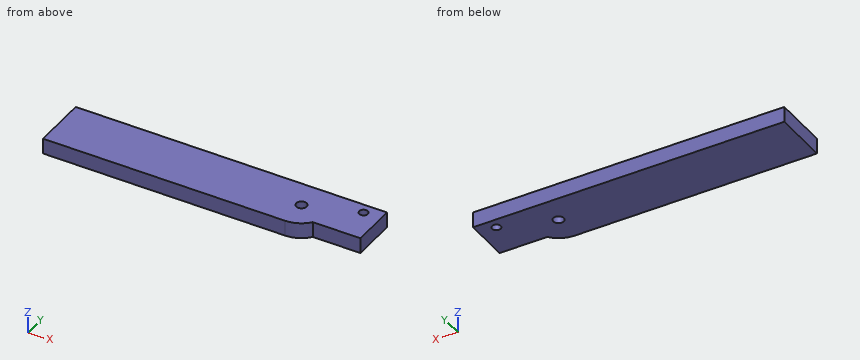
```python
from build123d import *

# Parameters (mm, degrees)
F1_DEPTH = 4.5
F2_D     = 3
F2_DEPTH = 10
F2_TIP   = 0.9012909285
F3_D     = 2.5
F3_DEPTH = 10
F3_TIP   = 0.7510757738


with BuildPart() as f1:
    # F0 (on Top) → F1 (new body)
    with BuildSketch(Plane.XY):
        Polygon((35, -5), (35, 8), (-35, 8), (-35, -8), (35, -8), align=None)
        with BuildLine():
            Line((41.2449979984, -5), (35, -5))
            Line((35, -5), (35, -8))
            ThreePointArc((35, -8), (38.4641016151, -7.2111025509), (41.2449979984, -5))
        make_face()
        with BuildLine():
            ThreePointArc((41.2449979984, -5), (42.2111025509, 3.4641016151), (35, 8))
            Line((35, 8), (35, -5))
            Line((35, -5), (41.2449979984, -5))
        make_face()
        with BuildLine():
            Line((55, 8), (35, 8))
            ThreePointArc((35, 8), (42.2111025509, 3.4641016151), (41.2449979984, -5))
            Line((41.2449979984, -5), (55, -5))
            Line((55, -5), (55, 8))
        make_face()
    extrude(amount=F1_DEPTH)

    # F2
    with Locations(Plane(origin=(0, 0, 0), x_dir=(1, 0, 0), z_dir=(0, 0, -1))):
        with Locations((35, 0)):
            Hole(F2_D / 2, depth=F2_DEPTH)
            with Locations((0, 0, -(F2_DEPTH + F2_TIP / 2))):  # 118° drill point
                Cone(0, F2_D / 2, F2_TIP, mode=Mode.SUBTRACT)

    # F3
    with Locations(Plane(origin=(0, 0, 0), x_dir=(1, 0, 0), z_dir=(0, 0, -1))):
        with Locations((50, -5)):
            Hole(F3_D / 2, depth=F3_DEPTH)
            with Locations((0, 0, -(F3_DEPTH + F3_TIP / 2))):  # 118° drill point
                Cone(0, F3_D / 2, F3_TIP, mode=Mode.SUBTRACT)


solid = f1.part
```
Model file for the job. Use its own axes, mm. Give positions to 0.01 mm unless a question says otherwise; leave off trailing zeros. Loops run counter-clockwise (first coordinate to the right, second up) from the corner with the lowest first, then second, coordinate; pieces in that order, holes last. Notation, with made-up numbers: M 6.5,32.5 L 56.5,32.5 A11 cw 56.5,53.5 Z; hole C 68,83 d9. An arc over 180 degrees is marked long. Use one line per item in the form item = value.
Item 1: Slice it at A-A on y = 0. List the corners of the cut face in (x, z), and give its area (4 significant figures).
Filled in:
outline = M -35,0 L 33.5,0 L 33.5,4.5 L -35,4.5 Z; M 36.5,0 L 55,0 L 55,4.5 L 36.5,4.5 Z
area = 391.5 mm^2
Item 2: Drill centre lines: L1, parallel to Y at x = 50, z = 2.8; L2, parallel to X at y = 5, z = 2.7; L3, parallel to Y at x = 35, z = 1.65. Where is each one in solid material? Low to high.
Filled in:
L1 = -5 to 3.75, 6.25 to 8
L2 = -35 to 48.75, 51.25 to 55
L3 = -8 to -1.5, 1.5 to 8
Item 3: Slice it at B-B on x = 50. List the corners of the cut face in (y, z).
Filled in:
outline = M -5,0 L 3.75,0 L 3.75,4.5 L -5,4.5 Z; M 6.25,0 L 8,0 L 8,4.5 L 6.25,4.5 Z
Item 4: Slice it at C-C on z = 2. List the corners of the cut face in (x, y) (3 decimals), and give its area (3 significant figures).
Filled in:
outline = M -35,-8 L 35,-8 A8 ccw 41.245,-5 L 55,-5 L 55,8 L -35,8 Z; hole C 35,0 d3; hole C 50,5 d2.5
area = 1,380 mm^2
Item 5: Flat gauge pins, fed straight in: pin 1 Ø2 at (x, y) = (50, 5) entering from -Z; pin 2 Ø5 at (x, y) = (-11.5, 6) entering from -Z; pin 3 Ø1.3 at (x, z) = (51.5, 2) entering from -Y. Where does each tip first touch, or does it go through?
Filled in:
pin_1 = through
pin_2 = 0
pin_3 = -5
Item 6: Slice it at D-D on y = -6.75. List the corners of the cut face in (x, z).
Filled in:
outline = M -35,0 L 39.29,0 L 39.29,4.5 L -35,4.5 Z
